from build123d import *

# Parameters (mm, degrees)
F0_W      = 17
F0_H      = 25
F1_DEPTH  = 3.25
F3_DEPTH  = 29
F4_R      = 2
F5_R      = 2
F6_R      = 2
F7_R      = 2
F8_R      = 0.907486
F8_R_2    = 0.912689
F9_DEPTH  = 1.13
F11_DEPTH = 0.41
F12_R     = 0.75
F13_DEPTH = 0.14
F15_DEPTH = 0.63
F17_DEPTH = 0.1


with BuildPart() as f1:
    # F0 (on Top) → F1 (new body, symmetric)
    with BuildSketch(Plane.XY):
        Rectangle(F0_W, F0_H)
    extrude(amount=F1_DEPTH, both=True)

    # F2 (on face) → F3 (cut)
    with BuildSketch(Plane.XZ.offset(12.5)):
        with BuildLine():
            Line((-3.064445, -3.25), (0, -3.25))
            ThreePointArc((0, -3.25), (-1.532222, -2.787639), (-3.064445, -3.25))
        make_face()
    extrude(amount=-F3_DEPTH, mode=Mode.SUBTRACT)

    # F4
    f4_edges = [f1.edges().sort_by_distance(p)[0] for p in [
        (0, -12.5, 3.25),
    ]]
    fillet(f4_edges, radius=F4_R)

    # F5
    f5_edges = [f1.edges().sort_by_distance(p)[0] for p in [
        (0, 12.5, 3.25),
    ]]
    fillet(f5_edges, radius=F5_R)

    # F6
    f6_edges = [f1.edges().sort_by_distance(p)[0] for p in [
        (8.5, 0, 3.25),
    ]]
    fillet(f6_edges, radius=F6_R)

    # F7
    f7_edges = [f1.edges().sort_by_distance(p)[0] for p in [
        (8.5, 0, -3.25),
    ]]
    fillet(f7_edges, radius=F7_R)

    # F8 (on face) → F9 (cut)
    with BuildSketch(Plane.YZ.offset(8.5)):
        with Locations((-10.477439, 0)):
            Circle(F8_R)
        with Locations((10.476667, 0)):
            Circle(F8_R_2)
    extrude(amount=-F9_DEPTH, mode=Mode.SUBTRACT)

    # F10 (on face) → F11 (cut)
    with BuildSketch(Plane.YZ.offset(8.5)):
        Polygon((6.696667, 1.843333), (-7.56, 1.82), (-8.4, -1.493333), (8.493334, -1.493333), align=None)
    extrude(amount=-F11_DEPTH, mode=Mode.SUBTRACT)

    # F12 (on face) → F13 (cut)
    with BuildSketch(Plane.YZ.offset(8.09)):
        with Locations((-6.826031, 0)):
            Circle(F12_R)
        with Locations((6.358803, 0)):
            Circle(F12_R)
    extrude(amount=-F13_DEPTH, mode=Mode.SUBTRACT)

    # F14 (on face) → F15 (cut)
    with BuildSketch(Plane.YZ.offset(8.09)):
        Polygon((-4.277901, 1.825372), (-5.225895, 1.82382), (-6.027778, -1.493333), (-5.104167, -1.493333), align=None)
        Polygon((-2.061455, 1.843333), (-2.989631, 1.82748), (-3.792398, -1.493333), (-2.868056, -1.493333), align=None)
        Polygon((0, 1.82), (-0.850787, 1.830981), (-1.654401, -1.493333), (-0.826389, -1.493333), align=None)
        Polygon((1.848753, 1.830981), (1.069426, 1.834123), (0.265052, -1.493333), (1.045139, -1.493333), align=None)
        Polygon((3.697775, 1.838425), (2.795116, 1.836948), (1.990059, -1.493333), (2.892361, -1.493333), align=None)
        Polygon((3.81221, -1.493333), (4.443903, -1.493333), (5.128974, 1.840768), (4.401408, 1.839577), align=None)
    extrude(amount=-F15_DEPTH, mode=Mode.SUBTRACT)

    # F16 (on face) → F17 (cut)
    with BuildSketch(Plane.XY.offset(3.25)):
        Polygon((-8.5, -4.322258), (6.5, -4.90492), (6.5, 5.395623), (-8.5, 5.621705), align=None)
    extrude(amount=-F17_DEPTH, mode=Mode.SUBTRACT)


solid = f1.part
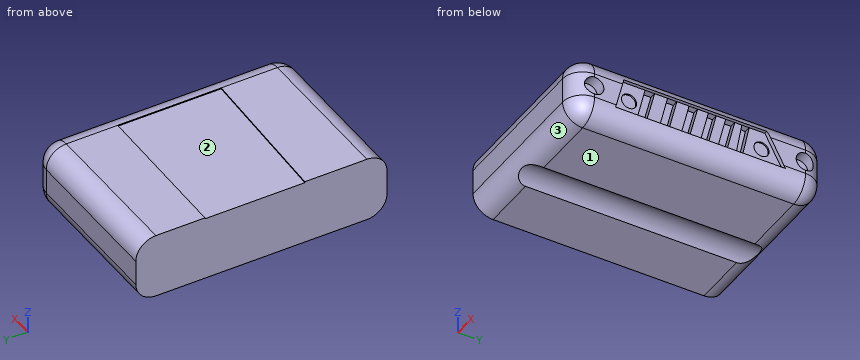
The listing builds one solid part. Answer for the finished solid, in the listing's coordinates (mm). Face numbers are marked on the shaded views. Give positions to 0.01 mm unless a question says otherwise; leave off trailing zeros. Write each loop counter-clockwise with the first axis right and the second up, starting at its lowest first coordinate (ties: lowest second). Pieces come first, ordered by that corner, then holes. Notation, with made-up numbers: (-37.75, 61) - (-33.75, 61) arc R28 cw to (-33.75, 86) - close; hole circle Ø1 at (-0.75, -36). An arc over 180 degrees is marked (long way). Use a Markdown table: item, result.
1. Section A-A on x = 1.75 is taken. Write down the section's boundary in (y, z), plus the area to 3 significant figures.
Values follow:
| item | result |
|---|---|
| outline | (-12.5, -1.25) arc R2 ccw to (-10.5, -3.25) - (10.5, -3.25) arc R2 ccw to (12.5, -1.25) - (12.5, 1.25) arc R2 ccw to (10.5, 3.25) - (5.47, 3.25) - (5.47, 3.15) - (-4.72, 3.15) - (-4.72, 3.25) - (-10.5, 3.25) arc R2 ccw to (-12.5, 1.25) - close |
| area | 158 mm² |
2. For a pull along Y with two mould halves and no side action, classify the marked faces 1, 2 and 3 as released by +Y, released by -Y, zero draft, split by the parting line, or undercut.
Values follow:
| item | result |
|---|---|
| face 1 | zero draft |
| face 2 | undercut |
| face 3 | released by -Y |
3. Each of these flat-tipped pins is pushed along its axis until it touches: P1, Ø1, axis at y = -7, z = 0.5, coming from the +X side; P2, Ø1.4, axis at y = 6.36, z = 0, coming from the +X side; P3, Ø1.1, axis at x = 7.5, y = 3.5, coming from the +Z side. Where does it stop, or does it pass through?
Values follow:
| item | result |
|---|---|
| P1 | stops at x = 8.09 |
| P2 | stops at x = 7.95 |
| P3 | stops at z = 3.2 |
4. Section B-B on y = -10 is taken. Write down the section's boundary in (x, z).
Values follow:
| item | result |
|---|---|
| outline | (-8.5, -3.25) - (-3.06, -3.25) arc R2.77 cw to (0, -3.25) - (6.5, -3.25) arc R2 ccw to (8.5, -1.25) - (8.5, -0.77) - (7.37, -0.77) - (7.37, 0.77) - (8.5, 0.77) - (8.5, 1.25) arc R2 ccw to (6.5, 3.25) - (-8.5, 3.25) - close |
5. Section C-C on z = -2 is taken. Write down the section's boundary in (x, y), plus the area to 3 significant figures.
Values follow:
| item | result |
|---|---|
| outline | (-8.5, -12.35) - (6.5, -12.35) arc R1.85 ccw to (8.35, -10.5) - (8.35, 10.5) arc R1.85 ccw to (6.5, 12.35) - (-8.5, 12.35) - close |
| area | 415 mm² |
6. Find the intervals of material crossed by probe 1 along Z at (x, y) = (1.5, -4.25); probe 2 along X at (y, z) = (-10.75, -1.75); probe 3 along Y at (x, z) = (4.5, -2.5), in increasing order. Write a range as from..to.
Values follow:
| item | result |
|---|---|
| probe 1 | z = -3.25..3.15 |
| probe 2 | x = -8.5..8.42 |
| probe 3 | y = -12.06..12.06 |
